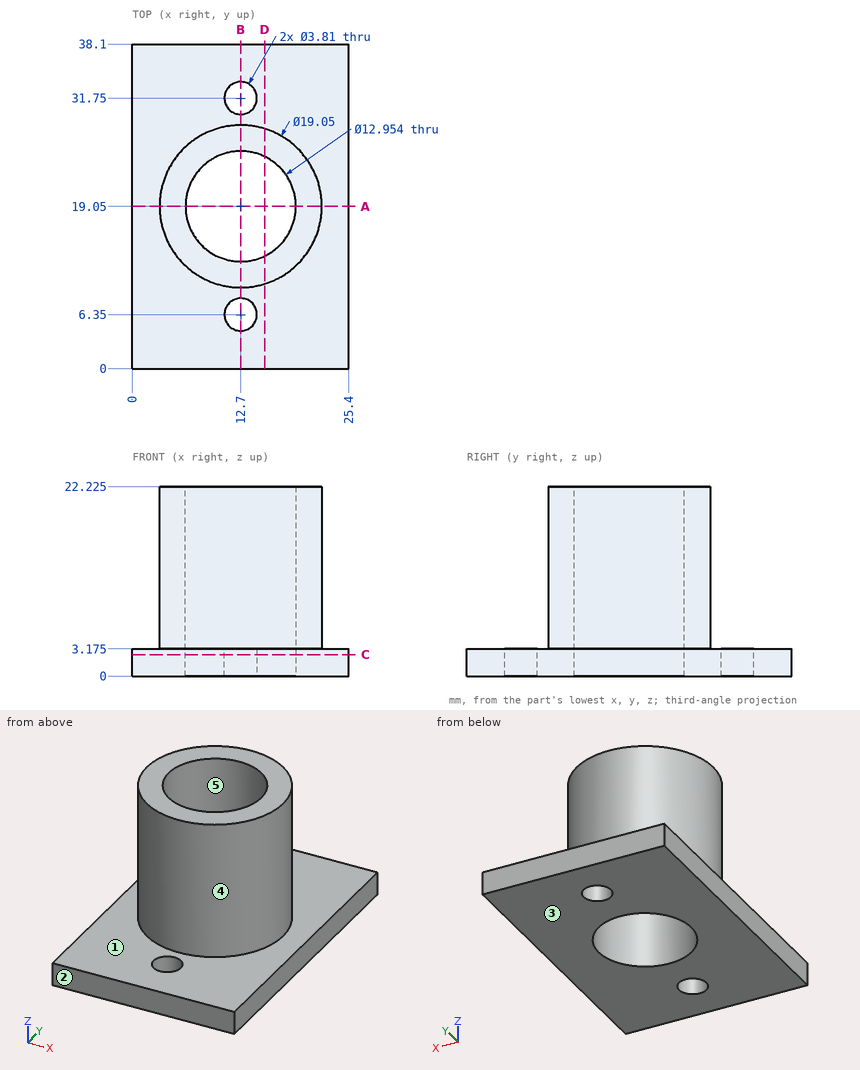
Can you work these out from the drawing? Everything is in mm from the part's minimum corner. A direction names the side the tool comes from. Round coordinates to 2 decimals unless told otherwise and drop trailing zeros. Order: outer loops, then holes, each group sorted by start corner. A loop starts at its lowest first (then second) coordinate and runs counter-clockwise, first axis right, second up. Notation, with made-up numbers: (77.5, 48.25) - (101.5, 48.25) arc R16 ccw to (101.5, 59.25) - close; hole circle Ø9 at (22, -5). An arc over 180 degrees is marked (long way). Answer in a Markdown table with one row per item.
(1) Suppose I cut it at B-B, the plane x = 12.7. Please give me the cut outline in (y, z) (3 decimals), plus the area to 3 significant figures.
From the geometry:
| item | result |
|---|---|
| outline | (0, 0) - (4.445, 0) - (4.445, 3.175) - (0, 3.175) - close; (8.255, 0) - (12.573, 0) - (12.573, 22.225) - (9.525, 22.225) - (9.525, 3.175) - (8.255, 3.175) - close; (25.527, 0) - (29.845, 0) - (29.845, 3.175) - (28.575, 3.175) - (28.575, 22.225) - (25.527, 22.225) - close; (33.655, 0) - (38.1, 0) - (38.1, 3.175) - (33.655, 3.175) - close |
| area | 172 mm2 |
(2) Please list where these lines run through material, in increasing order: L1, parallel to Y at x = 12.7, z = 1.15 (3 decimals); L2, parallel to X at y = 19, z = 10.5; L3, parallel to Y at x = 12.7, z = 7.25 (3 decimals). Write a range as from..to.
From the geometry:
| item | result |
|---|---|
| L1 | y = 0..4.445, 8.255..12.573, 25.527..29.845, 33.655..38.1 |
| L2 | x = 3.18..6.22, 19.18..22.22 |
| L3 | y = 9.525..12.573, 25.527..28.575 |
(3) If we mould it in two halves opening along X, with no side actions, what happens to the marked faces 3, 4 and 5? For each: released by +X, released by -X, zero draft, split by the parting line, or undercut.
From the geometry:
| item | result |
|---|---|
| face 3 | zero draft |
| face 4 | split by the parting line |
| face 5 | undercut |
(4) For P1, Ø12, axis at x = 19, z = 13, coming from the +Y side; P2, Ø6, axis at y = 15, z = 14, coming from the -X side; P3, Ø6, axis at x = 22, y = 5.5, coming from the +Z side (3 decimals), each with a flat end and sliding along its axis, tell me the tip position at first contact or that it passes through.
From the geometry:
| item | result |
|---|---|
| P1 | stops at y = 28.57 |
| P2 | stops at x = 3.23 |
| P3 | stops at z = 3.175 |
(5) Which directions (+Z, -Z, +X, -X, +Y, -Y) give clear straight access to the entire face, cutting with the end or side of a thin tool? Please do the marked faces 1 and 2.
From the geometry:
| item | result |
|---|---|
| face 1 | +Z |
| face 2 | +Z, -Z, +X, -X, -Y |
(6) Suppose I cut it at C-C, the plane z = 2.5. Please give me the cut outline in (x, y) (3 decimals), plus the area to 3 significant figures.
From the geometry:
| item | result |
|---|---|
| outline | (0, 0) - (25.4, 0) - (25.4, 38.1) - (0, 38.1) - close; hole circle Ø12.954 at (12.7, 19.05); hole circle Ø3.81 at (12.7, 6.35); hole circle Ø3.81 at (12.7, 31.75) |
| area | 813 mm2 |
(7) Suppose I cut it at A-A, the plane y = 19.05. Please give me the cut outline in (x, z) (3 decimals), plus the area to 3 significant figures.
From the geometry:
| item | result |
|---|---|
| outline | (0, 0) - (6.223, 0) - (6.223, 22.225) - (3.175, 22.225) - (3.175, 3.175) - (0, 3.175) - close; (19.177, 0) - (25.4, 0) - (25.4, 3.175) - (22.225, 3.175) - (22.225, 22.225) - (19.177, 22.225) - close |
| area | 156 mm2 |
(8) Suppose I cut it at D-D, the plane x = 15.5. Please give me the cut outline in (y, z) (1 decimal), plus the area to 3 significant figures.
From the geometry:
| item | result |
|---|---|
| outline | (0, 0) - (13.2, 0) - (13.2, 22.2) - (9.9, 22.2) - (9.9, 3.2) - (0, 3.2) - close; (24.9, 0) - (38.1, 0) - (38.1, 3.2) - (28.2, 3.2) - (28.2, 22.2) - (24.9, 22.2) - close |
| area | 208 mm2 |
